Design review of the part built by this model. Coordinates are the model's own, in mm. A direction names the side the tool comes from. Round coordinates to 2 decimals unless told otherwise and drop trailing zeros. Loops run counter-clockwise (first coordinate to the right, second up) from the corner with the lowest first, then second, coordinate; pieces in that order, holes last. Notation, with made-up numbers: (42.25, 11) - (55.25, 11) arc R31 cw to (55.25, 36) - close; hole circle Ø8 at (-26, -37). An arc over 180 degrees is marked (long way). Answer as CSV lines item,"result". Start each with the question number.
(1) Consider section C-C (y = -12.25). Give the boundary of the cut face in (x, z).
(2) Consider section B-B (x = 0). Give the boundary of the cut face in (y, z) (3 decimals).
(3) For faces 4 (the flat face through (-8.2, -15.875, 4.2)), 5 (the cylindrical face through (-9.219, -17.485, -8.784)), list the 3-axis set-ups (+Z, -Z, +X, -X, +Y, -Y) from which the entire face can be reached by the end or side of a thin tool; tool diameter is ignored.
(4) Consider section A-A (z = 0). Give the boundary of the cut face in (x, y) (3 decimals), and give its area (3 significant figures).
(5) Mouldability with a two-part tool opening along X and no side actions: class faces 1 (the cylindrical face through (8.633, -17.485, 9.911)), 2 (the cylindrical face through (-1.65, -7.2, -7.44)), 3 (the flat face through (0, -19.05, -8)) as released by +X, released by -X, zero draft, split by the parting line, or undercut.
(6) For P1, Ø2, axis at x = 10.5, z = -3.5, coming from the +Y side (3 decimals); P2, Ø10, axis at y = -7.5, z = 7.5, coming from the +X side; P3, Ø6, axis at y = -12.5, z = -1, coming from the -X side, all flat-tipped, find the tip position at first contact; note any pin that passes through.
(7) Wall thickness on L1, parallel to X at y = -17.5, z = 10.5; L2, parallel to Z at x = 3, y = -10.5; L3, parallel to Y at x = 8, z = -5 (3 decimals): over which ranges is each line inside the solid? List them lowest first.
from build123d import *

# Parameters (mm, degrees)
F0_R     = 7.62
F1_DEPTH = 19.05
F2_R     = 19.05
F2_R_2   = 7.62
F3_DEPTH = 3.175
F4_D     = 12.7
F5_R     = 1.27
F7_D     = 2.54


with BuildPart() as f1:
    # F0 (on Front) → F1 (new body)
    with BuildSketch(Plane.XZ):
        Circle(F0_R)
    extrude(amount=F1_DEPTH)

    # F2 (on face) → F3 (join)
    with BuildSketch(Plane.XZ.offset(19.05)):
        Circle(F2_R)
        Circle(F2_R_2, mode=Mode.SUBTRACT)
        Circle(F2_R_2)
    extrude(amount=-F3_DEPTH)

    # F4 (through all)
    with Locations(Plane(origin=(0, 0, 0), x_dir=(1, 0, 0), z_dir=(0, 1, 0))):
        with Locations((0, 0)):
            Hole(F4_D / 2)

    # F5
    f5_edges = [f1.edges().sort_by_distance(p)[0] for p in [
        (-19.05, -15.875, 0),
        (-7.62, -15.875, 0),
        (-19.05, -19.05, 0),
    ]]
    fillet(f5_edges, radius=F5_R)

    # F7 (through all)
    with Locations(Plane(origin=(0, -15.875, 0), x_dir=(-1, 0, 0), z_dir=(0, 1, 0))):
        with Locations((-9.90131, 9.8552), (9.8552, 9.90131), (9.90131, -9.8552), (-9.8552, -9.90131)):
            Hole(F7_D / 2)


solid = f1.part
Determined:
1,outline,"circle Ø15.24 at (0, 0); hole circle Ø12.7 at (0, 0)"
2,outline,"(-19.05, -17.78) arc R1.27 ccw to (-17.78, -19.05) - (-17.145, -19.05) arc R1.27 ccw to (-15.875, -17.78) - (-15.875, -8.89) arc R1.27 cw to (-14.605, -7.62) - (0, -7.62) - (0, -6.35) - (-19.05, -6.35) - close; (-19.05, 6.35) - (0, 6.35) - (0, 7.62) - (-14.605, 7.62) arc R1.27 cw to (-15.875, 8.89) - (-15.875, 17.78) arc R1.27 ccw to (-17.145, 19.05) - (-17.78, 19.05) arc R1.27 ccw to (-19.05, 17.78) - close"
3,face 4,"+Y"
3,face 5,"+Y, -Y"
4,outline,"(-19.05, -17.78) arc R1.27 ccw to (-17.78, -19.05) - (-6.35, -19.05) - (-6.35, 0) - (-7.62, 0) - (-7.62, -14.605) arc R1.27 cw to (-8.89, -15.875) - (-17.78, -15.875) arc R1.27 ccw to (-19.05, -17.145) - close; (6.35, -19.05) - (17.78, -19.05) arc R1.27 ccw to (19.05, -17.78) - (19.05, -17.145) arc R1.27 ccw to (17.78, -15.875) - (8.89, -15.875) arc R1.27 cw to (7.62, -14.605) - (7.62, 0) - (6.35, 0) - close"
4,area,"120 mm^2"
5,face 1,"undercut"
5,face 2,"split by the parting line"
5,face 3,"zero draft"
6,P1,"stops at y = -15.875"
6,P2,"stops at x = 7.2"
6,P3,"stops at x = -7.94"
7,L1,"x = -15.9 to -10.98, -8.74 to 8.81, 11 to 15.9"
7,L2,"z = -7 to -5.6, 5.6 to 7"
7,L3,"y = -19.05 to -15.875"
